Autodesk Inventor part; units mm, degrees
ref_plane "YZ Plane" through (0, 0, 0) normal (1, 0, 0) x (0, 1, 0)
ref_plane "XZ Plane" through (0, 0, 0) normal (0, 1, 0) x (-1, 0, 0)
ref_plane "XY Plane" through (0, 0, 0) normal (0, 0, 1) x (1, 0, 0)
sketch "スケッチ1" plane through (0, 0, 0) normal (0, 1, 0) x (-1, 0, 0)
  circle A0 centre (0, 0) radius 6
  circle A1 centre (0, 0) radius 4
  dimension "d0" = 12
  dimension "d1" = 8
extrude "押し出し1" add sketch "スケッチ1" along normal blind 3.5
sketch "スケッチ2" plane through (0, 3.5, 0) normal (0, 1, 0) x (1, 0, 0)
  circle A0 centre (0, 0) radius 6
  line L0 (-6, 0) -> (6, 0)
  line L1 (-6, 0.75) -> (6, 0.75)
  line L2 (-6, 0.75) -> (-6, 0)
  line L3 (6, 0.75) -> (6, 0)
  line L4 (-6, -0.75) -> (6, -0.75)
  line L5 (-6, -0.75) -> (-6, 0)
  line L6 (6, -0.75) -> (6, 0)
  point P0 (5.9529, 0.75)
  point P1 (-5.9529, 0.75)
  point P2 (-5.9529, -0.75)
  point P3 (5.9529, -0.75)
  dimension "d4" = 0.75
extrude "押し出し2" cut sketch "スケッチ2" against normal blind 0.3 contours L0 A0 L1 | A0 L4 L0
chamfer "面取り1" distance 0.3 angle 45 6 edges at (0, 3.5, 4) (0, 3.5, -4) (0, 3.5, -6) (0, 3.5, 6) (6, 0, 0) (4, 0, 0)
properties part number "GSB-081235"
Geometry check sheet. Reference: the model listing, model coordinates, mm. A direction names the side the tool comes from. Give positions to 0.01 mm unless a question says otherwise; leave off trailing zeros. Loops run counter-clockwise (first coordinate to the right, second up) from the corner with the lowest first, then second, coordinate; pieces in that order, holes last. Notation, with made-up numbers: (75, 74) -> (113, 74) arc R17 cw to (113, 79) -> close; hole circle Ø2 at (-21, 65.25). An arc over 180 degrees is marked (long way). Answer in a Markdown table with one row per item. Add a question column.
1) Gauge pin test, flat ends, axial feed: P1, Ø3, axis at x = 0, z = 1, coming from the -Y side; P2, Ø0.8, axis at x = 4.5, z = 0, coming from the +Y side; P3, Ø1, axis at x = -1.5, y = 3, coming from the -Z side. Record the tip position at first contact, or that the pin passes through.
2) Cross-section at B-B on z = 0. Record the boundary of the cut face in (x, y).
3) Cross-section at C-C on y = 2.1. Record the boundary of the cut face in (x, z).
4) Material ranges on probe 1 along Z at (x, y) = (0, 1.85); probe 2 along X at (y, z) = (1.3, 1.25), recorded low to high. Write a range as from..to.
5) Set-up check for faces 1 (the face through (0.867, 1.73, 3.905)), 2 (the face through (0.08, 3.32, -4.12)), 3 (the face through (-5, 3.2, 0)): record each of +Z, -Z, +X, -X, +Y, -Y from which the full face is reachable in a straight line by a thin tool's end or side.
6) Cross-section at A-A on x = 0. Record the boundary of the cut face in (y, z), and give its area (3 significant figures).
7) Draft check along Z on faces 4 (the face through (0.4, 3.5, -4.5)), 5 (the face through (5, 3.2, 0)), 6 (the face through (0.12, 3.38, 5.82)). Enter one of: pulls with the +Z half, pulls with the -Z half, needs draft (parallel to the pull), parting line crosses it, or undercut.
Outcome:
| question | item | result |
|---|---|---|
| 1 | P1 | passes through |
| 1 | P2 | stops at y = 3.2 |
| 1 | P3 | stops at z = -5.92 |
| 2 | outline | (-6, 0.3) -> (-5.7, 0) -> (-4.3, 0) -> (-4, 0.3) -> (-4, 3.2) -> (-6, 3.2) -> close; (4, 0.3) -> (4.3, 0) -> (5.7, 0) -> (6, 0.3) -> (6, 3.2) -> (4, 3.2) -> close |
| 3 | outline | circle Ø12 at (0, 0); hole circle Ø8 at (0, 0) |
| 4 | probe 1 | z = -6..-4, 4..6 |
| 4 | probe 2 | x = -5.87..-3.8, 3.8..5.87 |
| 5 | face 1 | +Y, -Y |
| 5 | face 2 | +Y |
| 5 | face 3 | +X, -X, +Y |
| 6 | outline | (0, -5.7) -> (0.3, -6) -> (3.2, -6) -> (3.5, -5.7) -> (3.5, -4.3) -> (3.2, -4) -> (0.3, -4) -> (0, -4.3) -> close; (0, 4.3) -> (0.3, 4) -> (3.2, 4) -> (3.5, 4.3) -> (3.5, 5.7) -> (3.2, 6) -> (0.3, 6) -> (0, 5.7) -> close |
| 6 | area | 13.6 mm^2 |
| 7 | face 4 | needs draft |
| 7 | face 5 | undercut |
| 7 | face 6 | pulls with the +Z half |
